Geometry check sheet. Reference: the model listing, model coordinates, mm. A direction names the side the tool comes from. Coordinates: 2 decimals unless noted, no trailing zeros. Write each loop counter-clockwise with the first axis right and the second up, starting at its lowest first coordinate (ties: lowest second). Pieces come first, ordered by that corner, then holes. Notation, with made-up numbers: (-31, 13.25) -> (18, 13.25) arc R25 cw to (18, 34.25) -> close; hole circle Ø6 at (83, 53.25). An arc over 180 degrees is marked (long way). Use a Markdown table: item, result.
```python
from build123d import *

# Parameters (mm, degrees)
SKETCH1_R           = 76.2
SKETCH1_R_2         = 57.15
BOSS_EXTRUDE1_DEPTH = 6.35
SKETCH2_R           = 71.12
SKETCH2_R_2         = 62.23
BOSS_EXTRUDE2_DEPTH = 7.62
SKETCH4_R           = 1.905
CUT_EXTRUDE1_DEPTH  = 5.08
CIRPATTERN1_COUNT   = 6
SKETCH7_R           = 1.27
CUT_EXTRUDE2_DEPTH  = 2.54


with BuildPart() as part:
    # Sketch1 → Boss-Extrude1 (new body)
    with BuildSketch(Plane(origin=(0, 0, 0), x_dir=(1, 0, 0), z_dir=(0, 1, 0))):
        with Locations(Location((0, 0, 0), (0, 0, 270))):
            Circle(SKETCH1_R)
        with Locations(Location((0, 0, 0), (0, 0, 270))):
            Circle(SKETCH1_R_2, mode=Mode.SUBTRACT)
    extrude(amount=BOSS_EXTRUDE1_DEPTH)

    # Sketch2 → Boss-Extrude2 (add)
    with BuildSketch(Plane(origin=(0, 6.35, 0), x_dir=(1, 0, 0), z_dir=(0, 1, 0))):
        with Locations(Location((0, 0, 0), (0, 0, 90))):
            Circle(SKETCH2_R)
        with Locations(Location((0, 0, 0), (0, 0, 90))):
            Circle(SKETCH2_R_2, mode=Mode.SUBTRACT)
    extrude(amount=BOSS_EXTRUDE2_DEPTH)

    # Sketch4 → Cut-Extrude1 (cut)
    with BuildSketch(Plane.XY.offset(71.12)):
        with Locations((0, 10.16)):
            Circle(SKETCH4_R)
    cut_extrude1 = extrude(amount=-CUT_EXTRUDE1_DEPTH, mode=Mode.SUBTRACT)

    # CirPattern1: Cut-Extrude1 ×6 about axis
    cirpattern1_axis = Axis((0, 0, 0), (0, 1, 0))
    for i in range(1, CIRPATTERN1_COUNT):
        add(cut_extrude1.rotate(cirpattern1_axis, i * 360 / CIRPATTERN1_COUNT), mode=Mode.SUBTRACT)

    # Sketch7 → Cut-Extrude2 (cut)
    with BuildSketch(Plane(origin=(0, 6.35, 0), x_dir=(1, 0, 0), z_dir=(0, 1, 0))):
        with Locations(Location((37.1475, 64.341357374, 0), (0, 0, 270))):
            Circle(SKETCH7_R)
        with Locations(Location((74.295, 0, 0), (0, 0, 270))):
            Circle(SKETCH7_R)
        with Locations(Location((37.1475, -64.341357374, 0), (0, 0, 270))):
            Circle(SKETCH7_R)
        with Locations(Location((-37.1475, -64.341357374, 0), (0, 0, 270))):
            Circle(SKETCH7_R)
        with Locations(Location((-74.295, 0, 0), (0, 0, 270))):
            Circle(SKETCH7_R)
        with Locations(Location((-37.1475, 64.341357374, 0), (0, 0, 270))):
            Circle(SKETCH7_R)
    extrude(amount=-CUT_EXTRUDE2_DEPTH, mode=Mode.SUBTRACT)


solid = part.part
```
Item 1: Tool access check on faces 1 (the flat face through (57.18, 10.19, 33.04)), 2 (the flat face through (-50.4, 6.35, 50.4)), 3 (the flat face through (0, 10, -66.04)). Record the directions out of +Z, -Z, +X, -X, +Y, -Y that give a thin tool (end or side, any length) a straight path to the whole face; none if there is none.
Answer block:
| item | result |
|---|---|
| face 1 | none |
| face 2 | +Y |
| face 3 | -Z |
Item 2: Section check A-A on x = 0. Record the boundary of the cut face in (y, z) (3 decimals).
Answer block:
| item | result |
|---|---|
| outline | (0, -76.2) -> (6.35, -76.2) -> (6.35, -71.12) -> (8.255, -71.12) -> (8.255, -66.04) -> (12.065, -66.04) -> (12.065, -71.12) -> (13.97, -71.12) -> (13.97, -62.23) -> (6.35, -62.23) -> (6.35, -57.15) -> (0, -57.15) -> close; (0, 57.15) -> (6.35, 57.15) -> (6.35, 62.23) -> (13.97, 62.23) -> (13.97, 71.12) -> (12.065, 71.12) -> (12.065, 66.04) -> (8.255, 66.04) -> (8.255, 71.12) -> (6.35, 71.12) -> (6.35, 76.2) -> (0, 76.2) -> close |
Item 3: Section check D-D on z = 4. Record the boundary of the cut face in (x, y), then the cut area to 3 significant figures.
Answer block:
| item | result |
|---|---|
| outline | (-76.09, 0) -> (-57.01, 0) -> (-57.01, 6.35) -> (-62.1, 6.35) -> (-62.1, 13.97) -> (-71.01, 13.97) -> (-71.01, 6.35) -> (-76.09, 6.35) -> close; (57.01, 0) -> (76.09, 0) -> (76.09, 6.35) -> (71.01, 6.35) -> (71.01, 13.97) -> (62.1, 13.97) -> (62.1, 6.35) -> (57.01, 6.35) -> close |
| area | 378 mm^2 |
Item 4: Section check C-C on y = 10.16. Record the boundary of the cut face in (x, z) (3 decimals).
Answer block:
| item | result |
|---|---|
| outline | (-62.522, -33.897) -> (-58.145, -31.37) -> (-56.24, -34.67) -> (-60.617, -37.197) arc R71.12 ccw to (-1.905, -71.094) -> (-1.905, -66.04) -> (1.905, -66.04) -> (1.905, -71.094) arc R71.12 ccw to (60.617, -37.197) -> (56.24, -34.67) -> (58.145, -31.37) -> (62.522, -33.897) arc R71.12 ccw to (62.522, 33.897) -> (58.145, 31.37) -> (56.24, 34.67) -> (60.617, 37.197) arc R71.12 ccw to (1.905, 71.094) -> (1.905, 66.04) -> (-1.905, 66.04) -> (-1.905, 71.094) arc R71.12 ccw to (-60.617, 37.197) -> (-56.24, 34.67) -> (-58.145, 31.37) -> (-62.522, 33.897) arc R71.12 ccw to start; hole circle Ø124.46 at (0, 0) |
Item 5: Section check B-B on z = 21. Record the boundary of the cut face in (x, y), then the cut area to 3 significant figures.
Answer block:
| item | result |
|---|---|
| outline | (-73.25, 0) -> (-53.15, 0) -> (-53.15, 6.35) -> (-58.58, 6.35) -> (-58.58, 13.97) -> (-67.95, 13.97) -> (-67.95, 6.35) -> (-73.25, 6.35) -> close; (53.15, 0) -> (73.25, 0) -> (73.25, 6.35) -> (67.95, 6.35) -> (67.95, 13.97) -> (58.58, 13.97) -> (58.58, 6.35) -> (53.15, 6.35) -> close |
| area | 398 mm^2 |
Item 6: Mould release check, pull along Y, two halves, no side actions. Record for faces 4 (the flat face through (57, 0, 11)), 5 (the cylindrical face through (-60.374, 10.244, 32.66)), 6 (the cylindrical face through (-60.3, 9.43, -32.78)), 7 (the cylindrical face through (-46.367, 3.131, -60.47)): +Y half, -Y half, draft (parallel to the pull), parting line (faces both ways), or undercut.
Answer block:
| item | result |
|---|---|
| face 4 | -Y half |
| face 5 | undercut |
| face 6 | undercut |
| face 7 | draft |
Item 7: Thickness scan on L1, parallel to X at y = 5.8, z = 0 (3 decimals); L2, parallel to X at y = 6, z = -2 (3 decimals); L3, parallel to X at y = 11.25, z = 0. Record the ranges inside material, lowest first. Write a range as [from, to].
Answer block:
| item | result |
|---|---|
| L1 | x = [-76.2, -75.565], [-73.025, -57.15], [57.15, 73.025], [75.565, 76.2] |
| L2 | x = [-76.174, -57.115], [57.115, 76.174] |
| L3 | x = [-71.12, -62.23], [62.23, 71.12] |
Item 8: Depth check by flat-ended pin: P1, Ø1.1, axis at x = 1, y = 10, coming from the -Z side; P2, Ø1.3, axis at x = -75, z = 0, coming from the +Y side; P3, Ø4, axis at x = 49, y = 4.5, coming from the -Z side; P4, Ø1.5, axis at x = -37.15, z = 64.34, coming from the -Y side. Enter the tip coordinate at first touch or a pass-through.
Answer block:
| item | result |
|---|---|
| P1 | stops at z = -66.04 |
| P2 | stops at y = 6.35 |
| P3 | stops at z = -59.98 |
| P4 | stops at y = 0 |
